For this review, use the dimensioned drawing (mm, ordinates from the lowest corner) and the shaded views. Coordinates: 2 decimals unless noted, no trailing zeros. Loops run counter-clockwise (first coordinate to the right, second up) from the corner with the lowest first, then second, coordinate; pieces in that order, holes last. Notation, with made-up numbers: M 86,57 L 145,57 A29 ccw 145,93 Z; hole C -37,72 d6. An arc over 180 degrees is marked long. One line per item, written item: value.
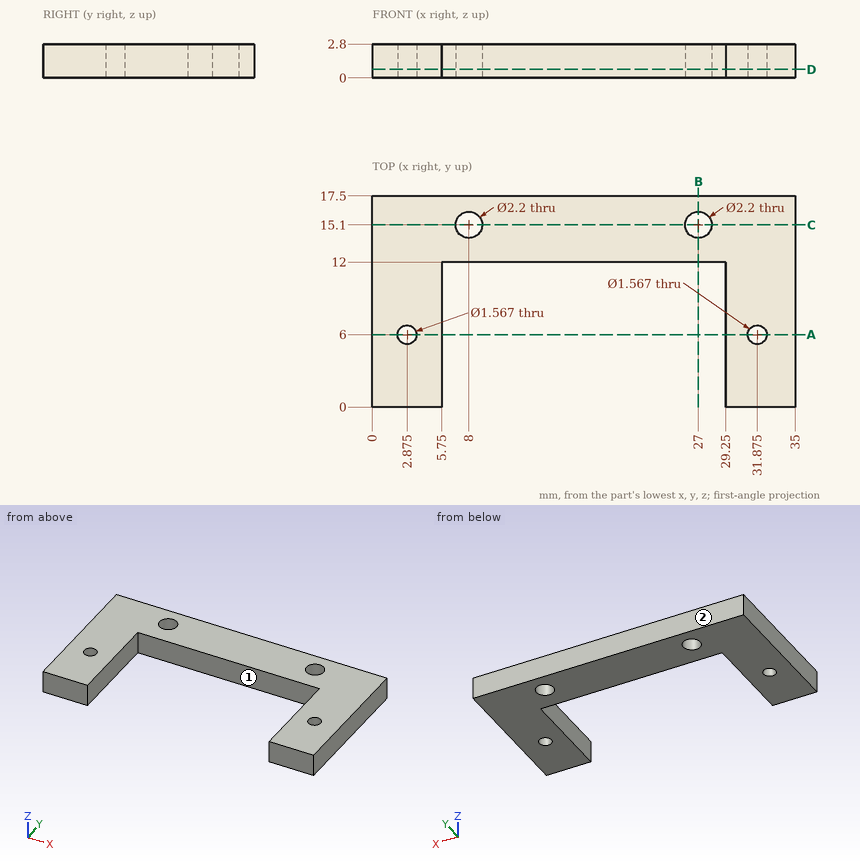
(1) Add section A-A on y = 6. State the section outline as (x, z) points.
Checks:
outline: M 0,0 L 2.09,0 L 2.09,2.8 L 0,2.8 Z; M 3.66,0 L 5.75,0 L 5.75,2.8 L 3.66,2.8 Z; M 29.25,0 L 31.09,0 L 31.09,2.8 L 29.25,2.8 Z; M 32.66,0 L 35,0 L 35,2.8 L 32.66,2.8 Z
(2) Insertion check: pin 1 Ø1.4 at (x, z) = (19, 1) entering from -Y. The pin has a flat end and moves straight along its axis. Give the tip position at first contact, or say it passes through.
Checks:
pin 1: y = 12
(3) To check wall thickness, follow L1, parallel to X at y = 6, z = 0.75; L2, parallel to X at y = 2, z = 0.7; L3, parallel to Y at x = 27, z = 1.05. State the ranges of each line that lie inside material, in increasing order. Write a range as [from, to].
Checks:
L1: [0, 2.09], [3.66, 5.75], [29.25, 31.09], [32.66, 35]
L2: [0, 5.75], [29.25, 35]
L3: [12, 14], [16.2, 17.5]
(4) Draft analysis for pull direction X (two halves, no side actions). For the marked faces 1 and 2, state which applies: pulls with the +X half, pulls with the -X half, needs draft (parallel to the pull), parting line crosses it, or undercut.
Checks:
face 1: undercut
face 2: needs draft
(5) Add section D-D on z = 0.7. State how many separate pieces and enclosed holes the cut face has, then the cut area to 3 significant figures.
Checks:
separate pieces: 1
enclosed holes: 4
area: 319 mm^2
(6) Add section C-C on y = 15.1. State the section outline as (x, z) points.
Checks:
outline: M 0,0 L 6.9,0 L 6.9,2.8 L 0,2.8 Z; M 9.1,0 L 25.9,0 L 25.9,2.8 L 9.1,2.8 Z; M 28.1,0 L 35,0 L 35,2.8 L 28.1,2.8 Z
(7) Add section B-B on x = 27. State the section outline as (y, z) points, then the cut area to 3 significant figures.
Checks:
outline: M 12,0 L 14,0 L 14,2.8 L 12,2.8 Z; M 16.2,0 L 17.5,0 L 17.5,2.8 L 16.2,2.8 Z
area: 9.24 mm^2
